from build123d import *

# Parameters (mm, degrees)
F0_W     = 88.9
F0_H     = 88.9
F1_DEPTH = 584.2
F2_W     = 88.9
F2_H     = 44.45
F3_DEPTH = 88.901
F5_DEPTH = 88.901


with BuildPart() as f1:
    # F0 (on Front) → F1 (new body)
    with BuildSketch(Plane.XZ):
        Rectangle(F0_W, F0_H)
    extrude(amount=-F1_DEPTH)

    # F2 (on face) → F3 (cut, through all)
    with BuildSketch(Plane.YZ.offset(44.45)):
        with Locations((44.45, 22.225)):
            Rectangle(F2_W, F2_H)
        with Locations((539.75, 22.225)):
            Rectangle(F2_W, F2_H)
    extrude(amount=-F3_DEPTH, mode=Mode.SUBTRACT)

    # F4 (on face) → F5 (cut, through all)
    with BuildSketch(Plane.YZ.offset(44.45)):
        Polygon((0, 0), (0, -44.45), (7.837734, 0), align=None)
    extrude(amount=-F5_DEPTH, mode=Mode.SUBTRACT)


solid = f1.part
Part model, mm, in its own coordinate system. A direction names the side the tool comes from. Give positions to 0.01 mm unless a question says otherwise; leave off trailing zeros. Order: outer loops, then holes, each group sorted by start corner. A loop starts at its lowest first (then second) coordinate and runs counter-clockwise, first axis right, second up. Notation, with made-up numbers: (-7.5, 59.25) -> (28.5, 59.25) arc R12 ccw to (28.5, 70.25) -> close; hole circle Ø6 at (26, -3). An arc over 180 degrees is marked (long way). Use one line per item in the form item = value.
(1) Tool access for faces 1 (the face through (-44.45, 288, -1)), 2 (the face through (1, 48, 0)), 3 (the face through (1, 539, 0)): list every direction of +Z, -Z, +X, -X, +Y, -Y with a clear straight run to the whole face (end or side of a thin tool).
Solution:
face_1 = +Z, -Z, -X, +Y, -Y
face_2 = +Z, +X, -X, -Y
face_3 = +Z, +X, -X, +Y
(2) Saw through at B-B (z = 22.5). Write the cut outline in (x, y), then the cut area to 3 significant figures.
Solution:
outline = (-44.45, 88.9) -> (44.45, 88.9) -> (44.45, 495.3) -> (-44.45, 495.3) -> close
area = 36,100 mm²
(3) Saw through at C-C (y = 546). Write the cut outline in (x, z).
Solution:
outline = (-44.45, -44.45) -> (44.45, -44.45) -> (44.45, 0) -> (-44.45, 0) -> close
(4) Drill centre lines: line 1 (Z direction, x = -30.5, y = 87); line 2 (Y direction, x = -25, z = 41). Where is each one in solid material? Low to high. Write a range as from..to.
Solution:
line_1 = -44.45..0
line_2 = 88.9..495.3
(5) Flat gauge pins, fed straight in: P1, Ø4, axis at x = -24.5, z = -27.5, coming from the -Y side; P2, Ø8, axis at x = -25.5, y = 500.5, coming from the +Z side; P3, Ø4, axis at x = -34, z = 7, coming from the +Y side. Where does each tip first touch, or does it go through?
Solution:
P1 = 2.64
P2 = 0
P3 = 495.3
(6) Saw through at A-A (x = 4.5). Write the cut outline in (y, z).
Solution:
outline = (0, -44.45) -> (584.2, -44.45) -> (584.2, 0) -> (495.3, 0) -> (495.3, 44.45) -> (88.9, 44.45) -> (88.9, 0) -> (7.84, 0) -> close
